Check sheet for the modelled part. Datum: model origin and axes. Units: mm. Give positions to 0.01 mm unless a question says otherwise; leave off trailing zeros. Order: outer loops, then holes, each group sorted by start corner. A loop starts at its lowest first (then second) coordinate and runs counter-clockwise, first axis right, second up.
from build123d import *

# Parameters (mm, degrees)
SKETCH3_W           = 40
SKETCH3_H           = 40
BOSS_EXTRUDE2_DEPTH = 5
BOSS_EXTRUDE3_DEPTH = 55


with BuildPart() as part:
    # Sketch3 → Boss-Extrude2 (new body, symmetric)
    with BuildSketch(Plane(origin=(0, 0, 0), x_dir=(1, 0, 0), z_dir=(0, 1, 0))):
        Rectangle(SKETCH3_W, SKETCH3_H)
    extrude(amount=BOSS_EXTRUDE2_DEPTH, both=True)

    # Sketch9 → Boss-Extrude3 (add, symmetric)
    with BuildSketch(Plane.XY):
        Polygon((-55, 5), (55, 5), (55, 152), (45, 152), (45, 15), (35, 15), (35, 152), (25, 152), (25, 15), (15, 15), (15, 152), (5, 152), (5, 15), (-5, 15), (-5, 152), (-15, 152), (-15, 15), (-25, 15), (-25, 152), (-35, 152), (-35, 15), (-45, 15), (-45, 152), (-55, 152), align=None)
    extrude(amount=BOSS_EXTRUDE3_DEPTH, both=True)


solid = part.part
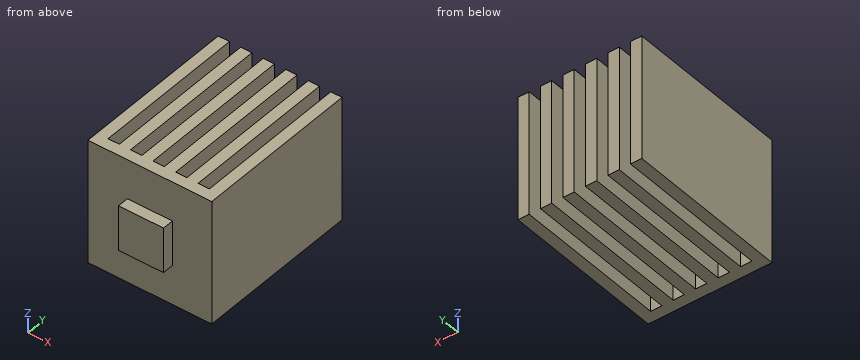
1) Section check D-D, the plane x = 8.5. Record the cut outline in (y, z), then the cut area to 3 significant figures.
Recorded:
outline: (-5, -20) - (5, -20) - (5, -55) - (152, -55) - (152, 55) - (5, 55) - (5, 20) - (-5, 20) - close
area: 16,600 mm2
2) Depth check by flat-ended pin: pin 1 Ø6 at (x, z) = (-39, 17.5) entering from -Y; pin 2 Ø5 at (x, z) = (19.5, -10.5) entering from +Y; pin 3 Ø8 at (y, z) = (0.5, -5.5) entering from -X; pin 4 Ø1.5 at (x, y) = (43.5, 44) entering from +Z. Enter the tip coordinate at first touch or a pass-through.
Recorded:
pin 1: stops at y = 5
pin 2: stops at y = 15
pin 3: stops at x = -20
pin 4: passes through
3) Section check C-C, the plane z = -8. Record the cut outline in (x, y), then the cut area to 3 significant figures.
Recorded:
outline: (-55, 5) - (-20, 5) - (-20, -5) - (20, -5) - (20, 5) - (55, 5) - (55, 152) - (45, 152) - (45, 15) - (35, 15) - (35, 152) - (25, 152) - (25, 15) - (15, 15) - (15, 152) - (5, 152) - (5, 15) - (-5, 15) - (-5, 152) - (-15, 152) - (-15, 15) - (-25, 15) - (-25, 152) - (-35, 152) - (-35, 15) - (-45, 15) - (-45, 152) - (-55, 152) - close
area: 9,720 mm2
4) Material ranges on L1, parallel to X at y = 66.5, z = -6; L2, parallel to Y at x = 22, z = -14; L3, parallel to Y at x = -2.5, z = 15, recorded low to high.
Recorded:
L1: x = -55 to -45, -35 to -25, -15 to -5, 5 to 15, 25 to 35, 45 to 55
L2: y = 5 to 15
L3: y = -5 to 15
5) Section check A-A, the plane y = 56. Record the cut outline in (x, z).
Recorded:
outline: (-55, -55) - (-45, -55) - (-45, 55) - (-55, 55) - close; (-35, -55) - (-25, -55) - (-25, 55) - (-35, 55) - close; (-15, -55) - (-5, -55) - (-5, 55) - (-15, 55) - close; (5, -55) - (15, -55) - (15, 55) - (5, 55) - close; (25, -55) - (35, -55) - (35, 55) - (25, 55) - close; (45, -55) - (55, -55) - (55, 55) - (45, 55) - close
6) Section check B-B, the plane x = -18. Record the cut outline in (y, z), then the cut area to 3 significant figures.
Recorded:
outline: (-5, -20) - (5, -20) - (5, -55) - (15, -55) - (15, 55) - (5, 55) - (5, 20) - (-5, 20) - close
area: 1,500 mm2
